from build123d import *

# Parameters (mm, degrees)
F1_DEPTH = 8
F2_R     = 0.99999


# Not quite as in the source:
# - a fillet or chamfer is up to 0.001 mm smaller than in the source, because OpenCascade refuses the exact size


with BuildPart() as f1:
    # F0 (on Top) → F1 (new body)
    with BuildSketch(Plane.XY):
        Polygon((20.5548869669, -26.5982374549), (20.5548869669, -18.3482374549), (22.3048869669, -18.3482374549), (22.3048869669, -26.5982374549), (23.3048869669, -26.5982374549), (23.3048869669, -18.3482374549), (23.3048869669, -8.3482374549), (22.3048869669, -8.3482374549), (22.3048869669, -16.5982374549), (20.5548869669, -16.5982374549), (20.5548869669, -8.3482374549), (19.5548869669, -8.3482374549), (19.5548869669, -18.3482374549), (19.5548869669, -26.5982374549), align=None)
    extrude(amount=F1_DEPTH)

    # F2 (radius 1 in the source; OpenCascade refuses exactly that, so slightly less here)
    f2_edges = [f1.edges().sort_by_distance(p)[0] for p in [
        (23.304887, -26.598237, 4),
        (23.304887, -17.473237, 8),
        (23.304887, -8.348237, 4),
        (23.304887, -17.473237, 0),
        (19.554887, -26.598237, 4),
        (19.554887, -17.473237, 8),
        (19.554887, -8.348237, 4),
        (19.554887, -17.473237, 0),
    ]]
    fillet(f2_edges, radius=F2_R)


solid = f1.part
Geometry check sheet. Reference: the model listing, model coordinates, mm. A direction names the side the tool comes from. Give positions to 0.01 mm unless a question says otherwise; leave off trailing zeros. Order: outer loops, then holes, each group sorted by start corner. A loop starts at its lowest first (then second) coordinate and runs counter-clockwise, first axis right, second up.
1) Material ranges on probe 1 along X at (y, z) = (-10, 6.75); probe 2 along Y at (x, z) = (20.85, 3); probe 3 along X at (y, z) = (-25.5, 0.5), recorded low to high.
Results are:
probe 1: x = 19.55 to 20.55, 22.3 to 23.3
probe 2: y = -18.35 to -16.6
probe 3: x = 19.69 to 20.55, 22.3 to 23.17
2) Tool access check on faces 5 (the cylindrical face through (19.84, -26.3, 4.06)), 6 (the flat face through (20.555, -13, 4)), 7 (the flat face through (21, -18.348, 4)). Record the directions out of +Z, -Z, +X, -X, +Y, -Y that give a thin tool (end or side, any length) a straight path to the whole face; none if there is none.
Results are:
face 5: +Z, -Z, -X, -Y
face 6: +Z, -Z, +Y
face 7: +Z, -Z, -Y
3) Gauge pin test, flat end, axial feed: pin 1 (0.9 mm diameter, centred on x = 21.5, z = 3, fed in from +Y). Record the tip position at first contact, or that the pin passes through.
Results are:
pin 1: stops at y = -16.6
4) Draft check along X on faces 1 (the flat face through (22.305, -22, 4)), 2 (the cylindrical face through (23.02, -17.35, 0.3)), 3 (the flat face through (20.555, -23, 4)), 4 (the cylindrical face through (19.84, -17.6, 0.3)). Enter one of: released by +X, released by -X, zero draft, split by the parting line, or undercut.
Results are:
face 1: undercut
face 2: released by +X
face 3: undercut
face 4: released by -X
5) Cross-section at C-C (y = -18). Record the boundary of the cut face in (x, z).
Results are:
outline: (19.55, 1) arc R1 ccw to (20.55, 0) - (22.3, 0) arc R1 ccw to (23.3, 1) - (23.3, 7) arc R1 ccw to (22.3, 8) - (20.55, 8) arc R1 ccw to (19.55, 7) - close
6) Cross-section at D-D (x = 20.85). Record the boundary of the cut face in (y, z), then the cut area to 3 significant figures.
Results are:
outline: (-18.35, 0) - (-16.6, 0) - (-16.6, 8) - (-18.35, 8) - close
area: 14.0 mm2
